For this review, take the finished solid that the model builds, in its own axes (mm). Give positions to 0.01 mm unless a question says otherwise; leave off trailing zeros. Loops run counter-clockwise (first coordinate to the right, second up) from the corner with the lowest first, then second, coordinate; pieces in that order, holes last.
```python
from build123d import *

# Parameters (mm, degrees)
SKETCH1_R                = 0.425
BOSS_EXTRUDE1_DEPTH      = 1.6
LPATTERN2_START          = -0.0125
LPATTERN2_OUTLINE_R      = 0.425
LPATTERN2_DEPTH          = 1.6
SLOTFOOTPRINTS_REF_DEPTH = 0.0001
SLOTFOOTPRINTS_DEPTH     = 0.0001
SKETCH2_R                = 0.8
F_20PIN_MOUNTS_DEPTH     = 71.235674696
SKETCH3_R                = 0.8
F_12PIN_MOUNTS_DEPTH     = 10


# Read off the part's stored shape, not the designer's step: LPattern2
with BuildPart() as part:
    # Sketch1 → Boss-Extrude1 (new body)
    with BuildSketch(Plane(origin=(0, 0, -0.0125), x_dir=(-1, 0, 0), z_dir=(0, 0, -1))):
        with BuildLine():
            Line((35.3, -50), (35.3, -48))
            ThreePointArc((35.3, -48), (35.592893219, -47.292893219), (36.3, -47))
            Line((36.3, -47), (45.8, -47))
            ThreePointArc((45.8, -47), (46.507106781, -46.707106781), (46.8, -46))
            Line((46.8, -46), (46.8, -41.4))
            ThreePointArc((46.8, -41.4), (47.092893219, -40.692893219), (47.8, -40.4))
            Line((47.8, -40.4), (49.3, -40.4))
            Line((49.3, -40.4), (49.3, 39.2))
            Line((49.3, 39.2), (43.2, 45.3))
            Line((43.2, 45.3), (35.500000002, 45.3))
            Line((35.500000002, 45.3), (3.499999998, 45.3))
            Line((3.499999998, 45.3), (-43.2, 45.3))
            Line((-43.2, 45.3), (-49.3, 39.2))
            Line((-49.3, 39.2), (-49.3, -40.4))
            Line((-49.3, -40.4), (-47.8, -40.4))
            ThreePointArc((-47.8, -40.4), (-47.092893219, -40.692893219), (-46.8, -41.4))
            Line((-46.8, -41.4), (-46.8, -46))
            ThreePointArc((-46.8, -46), (-46.507106781, -46.707106781), (-45.8, -47))
            Line((-45.8, -47), (-36.3, -47))
            ThreePointArc((-36.3, -47), (-35.592893219, -47.292893219), (-35.3, -48))
            Line((-35.3, -48), (-35.3, -50))
            Line((-35.3, -50), (35.3, -50))
        make_face()
        with Locations(Location((-21.27, 41.37, 0), (0, 0, 180))):
            Circle(SKETCH1_R, mode=Mode.SUBTRACT)
        with Locations(Location((-23.81, 41.37, 0), (0, 0, 180))):
            Circle(SKETCH1_R, mode=Mode.SUBTRACT)
        with Locations(Location((-22.54, 40.1, 0), (0, 0, 180))):
            Circle(SKETCH1_R, mode=Mode.SUBTRACT)
        with Locations(Location((-13.87, 41.37, 0), (0, 0, 180))):
            Circle(SKETCH1_R, mode=Mode.SUBTRACT)
        with Locations(Location((-23.81, 38.83, 0), (0, 0, 180))):
            Circle(SKETCH1_R, mode=Mode.SUBTRACT)
        with Locations(Location((-16.41, 41.37, 0), (0, 0, 180))):
            Circle(SKETCH1_R, mode=Mode.SUBTRACT)
        with Locations(Location((-15.14, 40.1, 0), (0, 0, 180))):
            Circle(SKETCH1_R, mode=Mode.SUBTRACT)
        with Locations(Location((-21.27, 38.83, 0), (0, 0, 180))):
            Circle(SKETCH1_R, mode=Mode.SUBTRACT)
        with Locations(Location((-28.67, 41.37, 0), (0, 0, 180))):
            Circle(SKETCH1_R, mode=Mode.SUBTRACT)
        with Locations(Location((-31.21, 41.37, 0), (0, 0, 180))):
            Circle(SKETCH1_R, mode=Mode.SUBTRACT)
        with Locations(Location((-16.41, 38.83, 0), (0, 0, 180))):
            Circle(SKETCH1_R, mode=Mode.SUBTRACT)
        with Locations(Location((-29.94, 40.1, 0), (0, 0, 180))):
            Circle(SKETCH1_R, mode=Mode.SUBTRACT)
        with Locations(Location((-31.21, 38.83, 0), (0, 0, 180))):
            Circle(SKETCH1_R, mode=Mode.SUBTRACT)
        with Locations(Location((-28.67, 38.83, 0), (0, 0, 180))):
            Circle(SKETCH1_R, mode=Mode.SUBTRACT)
        with Locations(Location((-13.87, 38.83, 0), (0, 0, 180))):
            Circle(SKETCH1_R, mode=Mode.SUBTRACT)
    extrude(amount=-BOSS_EXTRUDE1_DEPTH)

    # LPattern2 outline → LPattern2 (cut)
    with BuildSketch(Plane.XY.offset(LPATTERN2_START)):
        with Locations((31.21, 31.37)):
            Circle(LPATTERN2_OUTLINE_R)
        with Locations((31.21, 28.83)):
            Circle(LPATTERN2_OUTLINE_R)
        with Locations((29.94, 30.1)):
            Circle(LPATTERN2_OUTLINE_R)
        with Locations((28.67, 28.83)):
            Circle(LPATTERN2_OUTLINE_R)
        with Locations((28.67, 31.37)):
            Circle(LPATTERN2_OUTLINE_R)
        with Locations((16.41, 31.37)):
            Circle(LPATTERN2_OUTLINE_R)
        with Locations((23.81, 31.37)):
            Circle(LPATTERN2_OUTLINE_R)
        with Locations((23.81, 28.83)):
            Circle(LPATTERN2_OUTLINE_R)
        with Locations((22.54, 30.1)):
            Circle(LPATTERN2_OUTLINE_R)
        with Locations((21.27, 28.83)):
            Circle(LPATTERN2_OUTLINE_R)
        with Locations((21.27, 31.37)):
            Circle(LPATTERN2_OUTLINE_R)
        with Locations((16.41, 28.83)):
            Circle(LPATTERN2_OUTLINE_R)
        with Locations((15.14, 30.1)):
            Circle(LPATTERN2_OUTLINE_R)
        with Locations((13.87, 28.83)):
            Circle(LPATTERN2_OUTLINE_R)
        with Locations((13.87, 31.37)):
            Circle(LPATTERN2_OUTLINE_R)
    extrude(amount=LPATTERN2_DEPTH, mode=Mode.SUBTRACT)

    # thermalContacts_lower → slotFootprints_REF (cut)
    with BuildSketch(Plane(origin=(0, 0, -0.0125), x_dir=(-1, 0, 0), z_dir=(0, 0, -1))):
        Polygon((47, 35.5), (47, -41.5), (59.827263463, -41.5), (59.827263463, 47), (41.5, 47), (41.5, 41.5), (41.5, 35.5), align=None)
        Polygon((-47, 35.5), (-47, -41.5), (-56.192158269, -41.5), (-56.192158269, 47), (-41.5, 47), (-41.5, 41.5), (-41.5, 35.5), align=None)
    extrude(amount=-SLOTFOOTPRINTS_REF_DEPTH, mode=Mode.SUBTRACT)

    # thermalContacts_upper → slotFootprints (cut)
    with BuildSketch(Plane.XY.offset(1.5875)):
        Polygon((-47, 35.5), (-47, -41.5), (-56.192158269, -41.5), (-56.192158269, 47), (-41.5, 47), (-41.5, 41.5), (-41.5, 35.5), align=None)
        Polygon((47, 35.5), (47, -41.5), (59.827263463, -41.5), (59.827263463, 47), (41.5, 47), (41.5, 41.5), (41.5, 35.5), align=None)
    extrude(amount=-SLOTFOOTPRINTS_DEPTH, mode=Mode.SUBTRACT)

    # Sketch2 → 20pin_mounts (cut, through all)
    with BuildSketch(Plane.XY.offset(1.5875)):
        with Locations((-33.775, 38.472296419)):
            Circle(SKETCH2_R)
        with Locations((-17.925, 38.472296419)):
            Circle(SKETCH2_R)
        with Locations((-17.925, 28.472296419)):
            Circle(SKETCH2_R)
        with Locations((-33.775, 28.472296419)):
            Circle(SKETCH2_R)
        with BuildLine():
            Line((-35.775, 45.3), (-35.775, 43.8))
            ThreePointArc((-35.775, 43.8), (-35.482106781, 43.092893219), (-34.775, 42.8))
            Line((-34.775, 42.8), (-16.925, 42.8))
            ThreePointArc((-16.925, 42.8), (-16.217893218, 43.092893219), (-15.925, 43.8))
            Line((-15.925, 43.8), (-15.925, 45.3))
            Line((-15.925, 45.3), (-35.775, 45.3))
        make_face()
    extrude(amount=-F_20PIN_MOUNTS_DEPTH, mode=Mode.SUBTRACT)

    # Sketch3 → 12pin_mounts (cut)
    with BuildSketch(Plane(origin=(0, 0, -0.0125), x_dir=(-1, 0, 0), z_dir=(0, 0, -1))):
        with Locations((5.390000006, 41.4)):
            Circle(SKETCH3_R)
        with Locations((-5.379999994, 41.4)):
            Circle(SKETCH3_R)
    extrude(amount=-F_12PIN_MOUNTS_DEPTH, mode=Mode.SUBTRACT)


solid = part.part
```
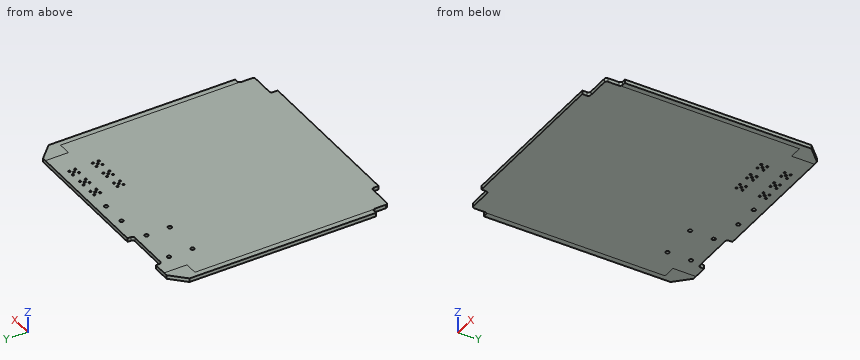
Q1. Consider section A-A on z = 1.15. Count the separate pieces of the cut face and the enclosed holes in it, plus the area to 3 significant figures.
Answers:
separate pieces: 1
enclosed holes: 36
area: 9,160 mm2
Q2. For probe 1 along Y at (x, z) = (31.21, 0.5) (3 decimals); probe 2 along Y at (x, z) = (-18, 0.85); probe 3 along X at (y, z) = (40.1, 1.3) (3 decimals), list the stretches that pass through material, from the lowest coordinate up.
Answers:
probe 1: y = -50 to 28.405, 29.255 to 30.945, 31.795 to 38.405, 39.255 to 40.945, 41.795 to 45.3
probe 2: y = -50 to 27.68, 29.27 to 37.68, 39.27 to 42.8
probe 3: x = -48.4 to 14.715, 15.565 to 22.115, 22.965 to 29.515, 30.365 to 48.4
Q3. Consider section B-B on x = -24.5. Give the boundary of the cut face in (y, z).
Answers:
outline: (-50, -0.01) - (42.8, -0.01) - (42.8, 1.59) - (-50, 1.59) - close
Q4. For pin 1 Ø0.8 at (x, z) = (-48, 0.5) entering from -Y; pin 2 Ø1.4 at (x, y) = (-17.92, 38.47) entering from +Z, all flat-tipped, find the tip position at first contact; note any pin that passes through.
Answers:
pin 1: stops at y = -40.42
pin 2: passes through
